The model under review builds one solid part; all positions refer to its coordinate system, in mm. Give positions to 0.01 mm unless a question says otherwise; leave off trailing zeros. Order: outer loops, then holes, each group sorted by start corner. A loop starts at its lowest first (then second) coordinate and runs counter-clockwise, first axis right, second up. Notation, with made-up numbers: (59, 78.5) - (83, 78.5) arc R20 cw to (83, 114.5) - close; hole circle Ø6 at (58.5, 80). An arc over 180 degrees is marked (long way). Put each result on its own line as item: value.
```python
from build123d import *

# Parameters (mm, degrees)
ESQUISSE1_W             = 41
ESQUISSE1_H             = 41
BOSS_EXTRU_1_DEPTH      = 0.3
ESQUISSE2_W             = 6
ESQUISSE2_H             = 4
BOSS_EXTRU_2_DEPTH      = 0.3
ESQUISSE3_R             = 12.5
ENL_V_MAT_EXTRU_1_DEPTH = 1.3
ESQUISSE4_R             = 16
ENL_V_MAT_EXTRU_2_DEPTH = 1.3
CHANFREIN1_SIZE         = 2
CHANFREIN2_SIZE         = 2
ESQUISSE6_W             = 6
ESQUISSE6_H             = 4
ENL_V_MAT_EXTRU_4_DEPTH = 1.3


with BuildPart() as part:
    # Esquisse1 → Boss.-Extru.1 (new body)
    with BuildSketch(Plane.XY):
        Rectangle(ESQUISSE1_W, ESQUISSE1_H)
    extrude(amount=BOSS_EXTRU_1_DEPTH)

    # Esquisse2 → Boss.-Extru.2 (add)
    with BuildSketch(Plane(origin=(0, 0, 0), x_dir=(-1, 0, 0), z_dir=(0, 0, -1))):
        with Locations((17.5, 22.5)):
            Rectangle(ESQUISSE2_W, ESQUISSE2_H)
        with Locations((-17.5, -22.5)):
            Rectangle(ESQUISSE2_W, ESQUISSE2_H)
        with Locations((17.5, -22.5)):
            Rectangle(ESQUISSE2_W, ESQUISSE2_H)
    extrude(amount=-BOSS_EXTRU_2_DEPTH)

    # Esquisse3 → Enlèv. mat.-Extru.1 (cut, through all)
    with BuildSketch(Plane(origin=(0, 0, 0), x_dir=(-1, 0, 0), z_dir=(0, 0, -1))):
        Circle(ESQUISSE3_R)
    extrude(amount=-ENL_V_MAT_EXTRU_1_DEPTH, mode=Mode.SUBTRACT)

    # Esquisse4 → Enlèv. mat.-Extru.2 (cut, through all)
    with BuildSketch(Plane(origin=(0, 0, 0), x_dir=(-1, 0, 0), z_dir=(0, 0, -1))):
        Circle(ESQUISSE4_R)
    extrude(amount=-ENL_V_MAT_EXTRU_2_DEPTH, mode=Mode.SUBTRACT)

    # Chanfrein1
    chanfrein1_edges = [part.edges().sort_by_distance(p)[0] for p in [
        (-20.5, -24.5, 0.15),
    ]]
    chamfer(chanfrein1_edges, length=CHANFREIN1_SIZE)

    # Chanfrein2
    chanfrein2_edges = [part.edges().sort_by_distance(p)[0] for p in [
        (20.5, -24.5, 0.15),
    ]]
    chamfer(chanfrein2_edges, length=CHANFREIN2_SIZE)

    # Esquisse6 → Enlèv. mat.-Extru.4 (cut, through all)
    with BuildSketch(Plane(origin=(0, 0, 0), x_dir=(-1, 0, 0), z_dir=(0, 0, -1))):
        with Locations((17.5, 22.5)):
            Rectangle(ESQUISSE6_W, ESQUISSE6_H)
    extrude(amount=-ENL_V_MAT_EXTRU_4_DEPTH, mode=Mode.SUBTRACT)


solid = part.part
```
(1) Wall thickness on L1, parallel to Y at x = 0, z = 0.1; L2, parallel to X at y = -0.5, z = 0.1; L3, parallel to X at y = 10, z = 0.05: over which ranges is each line inside the solid? List them lowest first.
The answers:
L1: -20.5 to -16, 16 to 20.5
L2: -20.5 to -15.99, 15.99 to 20.5
L3: -20.5 to -12.49, 12.49 to 20.5
(2) Take a section at A-A, the plane z = 0.1. Write out the cut boundary in (x, y), then the cut area to 3 significant figures.
The answers:
outline: (-20.5, -22.5) - (-18.5, -24.5) - (-14.5, -24.5) - (-14.5, -20.5) - (14.5, -20.5) - (14.5, -24.5) - (18.5, -24.5) - (20.5, -22.5) - (20.5, 20.5) - (-20.5, 20.5) - close; hole circle Ø32 at (0, 0)
area: 921 mm^2
(3) Take a section at B-B, the plane x = 0. Write out the cut boundary in (y, z).
The answers:
outline: (-20.5, 0) - (-16, 0) - (-16, 0.3) - (-20.5, 0.3) - close; (16, 0) - (20.5, 0) - (20.5, 0.3) - (16, 0.3) - close
